from build123d import *

# Parameters (mm, degrees)
SKETCH1_R               = 10
BOSS_EXTRUDE1_DEPTH     = 9.5
CUT_EXTRUDE3_DEPTH      = 25
CUT_EXTRUDE3_DEPTH_BACK = 25
SKETCH3_R               = 1.65
CUT_EXTRUDE4_DEPTH      = 25
CUT_EXTRUDE4_DEPTH_BACK = 25
SKETCH4_R               = 1.65
BOSS_EXTRUDE3_START     = 5
SKETCH6_R               = 10
BOSS_EXTRUDE3_DEPTH     = 5
CUT_EXTRUDE1_DEPTH      = 25
BOSS_EXTRUDE4_DEPTH     = 5
FILLET1_R               = 3
CUT_EXTRUDE5_DEPTH      = 100
CUT_EXTRUDE5_DEPTH_BACK = 100
SKETCH8_R               = 1.65


with BuildPart() as part:
    # Sketch1 → Boss-Extrude1 (new body)
    with BuildSketch(Plane(origin=(0, 0, 0), x_dir=(0, 0, -1), z_dir=(1, 0, 0))):
        Circle(SKETCH1_R)
    extrude(amount=BOSS_EXTRUDE1_DEPTH)

    # Sketch3 → Cut-Extrude3 (cut, two sides: drawn at the far end of the back side and taken through both)
    with BuildSketch(Plane(origin=(0, 0, 0), x_dir=(1, 0, 0), z_dir=(0, 1, 0)).offset(-CUT_EXTRUDE3_DEPTH_BACK)):
        with Locations((1.5, 0)):
            Circle(SKETCH3_R)
    extrude(amount=CUT_EXTRUDE3_DEPTH + CUT_EXTRUDE3_DEPTH_BACK, mode=Mode.SUBTRACT)

    # Sketch4 → Cut-Extrude4 (cut, two sides: drawn at the far end of the back side and taken through both)
    with BuildSketch(Plane.XY.offset(-CUT_EXTRUDE4_DEPTH_BACK)):
        with Locations((1.5, 0)):
            Circle(SKETCH4_R)
    extrude(amount=CUT_EXTRUDE4_DEPTH + CUT_EXTRUDE4_DEPTH_BACK, mode=Mode.SUBTRACT)

    # Sketch6 → Boss-Extrude3 (add)
    with BuildSketch(Plane.ZY.offset(BOSS_EXTRUDE3_START)):
        Circle(SKETCH6_R)
    extrude(amount=-BOSS_EXTRUDE3_DEPTH)

    # Sketch2 → Cut-Extrude1 (cut)
    with BuildSketch(Plane.ZY.offset(-9.5)):
        with BuildLine():
            ThreePointArc((2.6, 0), (2.353661446, 1.104661847), (1.661324773, 2))
            Line((1.661324773, 2), (-1.661324773, 2))
            ThreePointArc((-1.661324773, 2), (-1.104661847, -2.353661446), (2.6, 0))
        make_face()
    extrude(amount=CUT_EXTRUDE1_DEPTH, mode=Mode.SUBTRACT)

    # Sketch7 → Boss-Extrude4 (add)
    with BuildSketch(Plane.ZY.offset(5)):
        Polygon((-3, -5.196152423), (3, -5.196152423), (6, 0), (3, 5.196152423), (-3, 5.196152423), (-6, 0), align=None)
        Polygon((1.732050808, -3), (3.464101615, 0), (1.732050808, 3), (-1.732050808, 3), (-3.464101615, 0), (-1.732050808, -3), align=None, mode=Mode.SUBTRACT)
    extrude(amount=BOSS_EXTRUDE4_DEPTH)

    # Fillet1
    fillet1_edges = [part.edges().sort_by_distance(p)[0] for p in [
        (-5, -2.598076211, -4.5),
        (-5, -5.196152423, 0),
        (-5, -2.598076211, 4.5),
        (-5, 2.598076211, 4.5),
        (-5, 5.196152423, 0),
        (-5, 2.598076211, -4.5),
    ]]
    fillet(fillet1_edges, radius=FILLET1_R)

    # Sketch8 → Cut-Extrude5 (cut, two sides: drawn at the far end of the back side and taken through both)
    with BuildSketch(Plane(origin=(0, -5.196152423, 0), x_dir=(-1, 0, 0), z_dir=(0, -1, 0)).offset(-CUT_EXTRUDE5_DEPTH_BACK)):
        with Locations(Location((7.5, 0, 0), (0, 0, 287.639701394))):
            Circle(SKETCH8_R)
    extrude(amount=CUT_EXTRUDE5_DEPTH + CUT_EXTRUDE5_DEPTH_BACK, mode=Mode.SUBTRACT)


solid = part.part
Work out the finished part from the listing and answer in its coordinate system (mm). A direction names the side the tool comes from. Coordinates: 2 decimals unless noted, no trailing zeros. Write each loop counter-clockwise with the first axis right and the second up, starting at its lowest first coordinate (ties: lowest second). Pieces come first, ordered by that corner, then holes. Notation, with made-up numbers: M -37.75,40.5 L -8.75,40.5 A17 ccw -8.75,66.5 Z; hole C 37,-38.5 d2. An arc over 180 degrees is marked long. Answer as CSV lines item,"result". Start each with the question number.
Item 1: Section C-C on x = 6.75 is taken. Write down the section's boundary in (y, z).
Item 2: Determine the mould class of faces 6 (the face through (-5.52, -3.31, -5.6)), 7 (the face through (0, 0, -6)), 8 (the face through (4, 2, 0)) for opening direction X: released by +X, released by -X, zero draft, split by the parting line, or undercut.
Item 3: Flat-ended cylindrical pins translate along their axes: P1, Ø4.5, axis at x = 1.5, z = 0, coming from the +Y side; P2, Ø1.5, axis at x = 1.5, z = 4.5, coming from the +Y side; P3, Ø3, axis at x = -7.5, z = 0, coming from the +Y side (3 decimals); P4, Ø1, axis at x = -1.5, y = -3.5, coming from the -Z side. Find the tip coordinate at first contact, or state that the pin passes through.
Item 4: A tool of negligible diameter and unlimited length cuts with its end or side. For faces 1 (the face through (-9, 2.6, -4.5)), 2 (the face through (0, 0, 6)), 3 (the face through (-5, 3.8, -7.5)), 4 (the face through (0, -6, 0)), 5 (the face through (-9, -2.6, 4.5)), from which of +Z, -Z, +X, -X, +Y, -Y can it reach the whole face along a straight path? Write none if from no direction.
Item 5: Section A-A on z = 0 is taken. Give the number of separate pieces and of enclosed holes in the cut face, and give its area (3 significant figures).
Item 6: Consider L1, parallel to X at y = 0, z = -5.25; L2, parallel to X at y = 4.05, z = 0; L3, parallel to X at y = 5.5, z = 0. Determine where each line is inside the solid, lowest interval first.
Item 7: Section B-B on x = -7.5 is taken. Write down the section's boundary in (y, z), and give its area (3 significant figures).
Checks:
1,outline,"C 0,0 d20; hole M 2,-1.66 L 2,1.66 A2.6 ccw long Z"
2,face 6,"released by -X"
2,face 7,"undercut"
2,face 8,"zero draft"
3,P1,"stops at y = 10"
3,P2,"stops at y = 9.27"
3,P3,"passes through"
3,P4,"stops at z = -9.54"
4,face 1,"-Z, -X, +Y"
4,face 2,"+Z, -Z"
4,face 3,"-X"
4,face 4,"+Y, -Y"
4,face 5,"+Z, -X, -Y"
5,separate pieces,"6"
5,enclosed holes,"0"
5,area,"185 mm²"
6,L1,"x = -10 to 0, 3.15 to 9.5"
6,L2,"x = -10 to -9.15, -5.85 to 0, 3.15 to 9.5"
6,L3,"x = -5.85 to 0, 3.15 to 9.5"
7,outline,"M -5.24,-3.02 L 0,-6.05 L 5.24,-3.02 L 5.24,-1.65 L 3,-1.65 L 3,-1.73 L 0,-3.46 L -3,-1.73 L -3,-1.65 L -5.24,-1.65 Z; M -5.24,1.65 L -3,1.65 L -3,1.73 L 0,3.46 L 3,1.73 L 3,1.65 L 5.24,1.65 L 5.24,3.02 L 0,6.05 L -5.24,3.02 Z"
7,area,"49.1 mm²"
